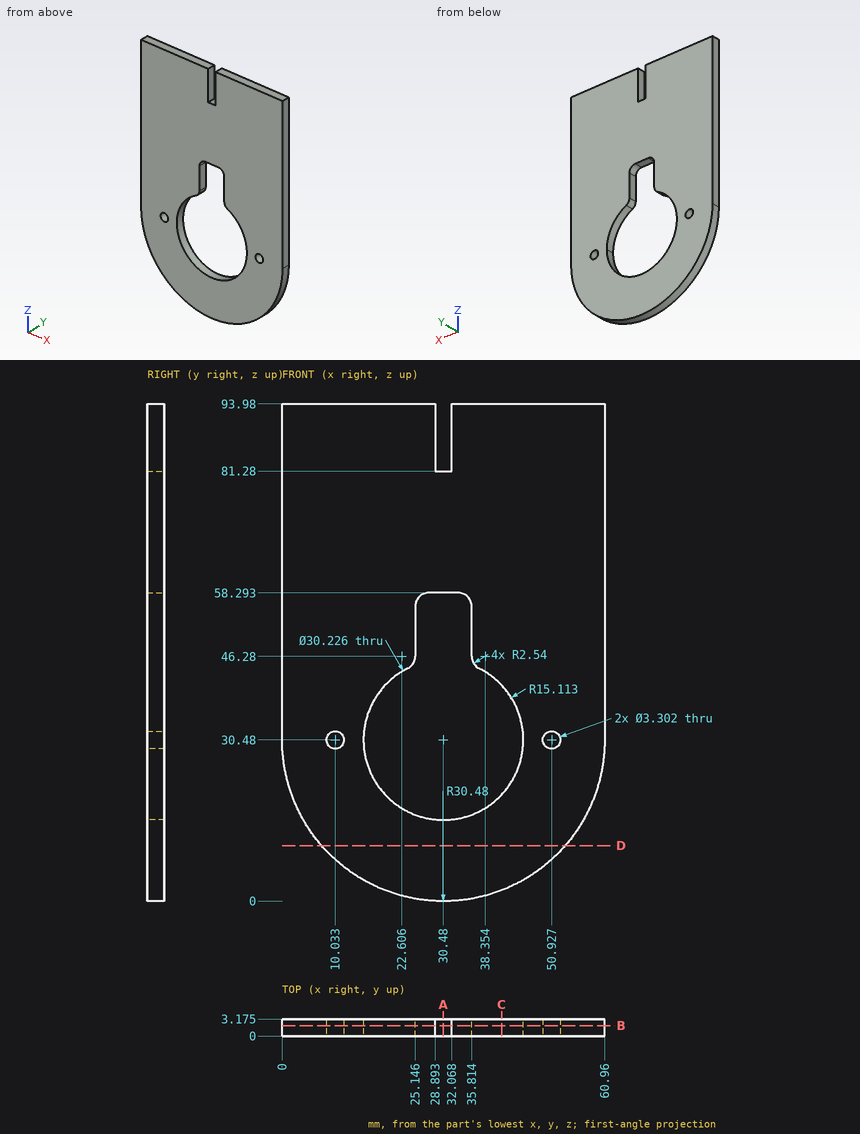
Input: dimensioned drawing with shaded views. Units: mm. Origin: part minimum x, y, z. Give positions to 0.01 mm unless a question says otherwise; leave off trailing zeros. Write each loop counter-clockwise with the first axis right and the second up, starting at its lowest first coordinate (ties: lowest second). Pieces come first, ordered by that corner, then holes. Notation, with made-up numbers: (17, 0) -> (68, 0) arc R11 ccw to (68, 9) -> close; hole circle Ø8 at (37, -40). An arc over 180 degrees is marked (long way). Answer as a JSON object with one key per item and string values.
1. Cut plane C-C on x = 41.5. Output: boundary loops of the cut face in (y, z) (1 decimal).
Ans:
{"outline": "(0, 2.1) -> (3.2, 2.1) -> (3.2, 20.1) -> (0, 20.1) -> close; (0, 40.8) -> (3.2, 40.8) -> (3.2, 94) -> (0, 94) -> close"}
2. Cut plane A-A on x = 30.48. Output: boundary loops of the cut face in (y, z) (1 decimal).
Ans:
{"outline": "(0, 0) -> (3.2, 0) -> (3.2, 15.4) -> (0, 15.4) -> close; (0, 58.3) -> (3.2, 58.3) -> (3.2, 81.3) -> (0, 81.3) -> close"}
3. Cut plane D-D on z = 10.5. Output: boundary loops of the cut face in (x, y) (1 decimal), and give its area (3 significant figures).
Ans:
{"outline": "(7.5, 0) -> (53.5, 0) -> (53.5, 3.2) -> (7.5, 3.2) -> close", "area": "146 mm^2"}
4. Ray query, probe 1 along X at (y, z) = (0.55, 48.5) (1 decimal); probe 2 along X at (y, z) = (2.4, 29) (1 decimal); probe 3 along X at (y, z) = (2.95, 37.5) (1 decimal). Return the intervals inside material, ascending. Write a range as from..to.
Ans:
{"probe 1": "x = 0..25.1, 35.8..61", "probe 2": "x = 0..9.3, 10.8..15.4, 45.5..50.2, 51.7..60.9", "probe 3": "x = 0..17.1, 43.9..61"}
5. Cut plane B-B on y = 1.95. Count the separate pieces of the cut face and the enclosed holes in it, and give its area (3 significant figures).
Ans:
{"separate pieces": "1", "enclosed holes": "3", "area": "4,420 mm^2"}
6. Contact query for flat-ended pins moving along their axis: pin 1 (1 mm diameter, centred on x = 30, y = 2.5, fed in from +Z); pin 2 (1.5 mm diameter, centred on x = 17, y = 3, fed in from -Z) (1 decimal); pin 3 (1.6 mm diameter, centred on x = 31.5, y = 1.5, fed in from -Z). Output: stop coordinate, or through.
Ans:
{"pin 1": "stops at z = 81.28", "pin 2": "stops at z = 2.8", "pin 3": "stops at z = 0"}
